from build123d import *

# Parameters (mm, degrees)
F0_R     = 3
F1_DEPTH = 50
F2_R     = 1
F3_R     = 10
F3_R_2   = 3
F4_DEPTH = 20
F5_R     = 1


with BuildPart() as f1:
    # F0 (on Front) → F1 (new body)
    with BuildSketch(Plane.XZ):
        Circle(F0_R)
    extrude(amount=F1_DEPTH)

    # F2
    f2_edges = [f1.edges().sort_by_distance(p)[0] for p in [
        (-3, 0, 0),
    ]]
    fillet(f2_edges, radius=F2_R)

    # F3 (on face) → F4 (join)
    with BuildSketch(Plane.XZ.offset(50)):
        Circle(F3_R)
        Circle(F3_R_2, mode=Mode.SUBTRACT)
    extrude(amount=-F4_DEPTH)

    # F5
    f5_edges = [f1.edges().sort_by_distance(p)[0] for p in [
        (-3, -30, 0),
        (-10, -30, 0),
        (-10, -50, 0),
    ]]
    fillet(f5_edges, radius=F5_R)


solid = f1.part
Source: CAD feature listing. Evaluate the final solid. Frame: model axes, mm. A direction names the side the tool comes from. Coordinates: 2 decimals unless noted, no trailing zeros. Loops run counter-clockwise (first coordinate to the right, second up) from the corner with the lowest first, then second, coordinate; pieces in that order, holes last. Notation, with made-up numbers: (10, 20.25) -> (27, 20.25) arc R11 cw to (27, 32.25) -> close; hole circle Ø7 at (33, -29). An arc over 180 degrees is marked (long way). Answer in a Markdown table with one row per item. Add a question column.
Q1. Ray query, line 1 along Y through (x, z) = (-8, 0.5); line 2 along X through (y, z) = (-8.5, -0.25); line 3 along X through (y, z) = (-16.5, 1.5). Return the intervals inside material, ascending.
Q2. Section D-D on y = -27. Return the cut outline in (x, z).
Q3. Pull-direction query (Y, two-part tool) for faces 3 (the face through (0, -50, 0)), 4 (the face through (2, -30, -4)), 5 (the face through (-2.17, -40.13, -9.76)); classes: pulls with the +Y half, pulls with the -Y half, needs draft (parallel to the pull), parting line crosses it, or undercut.
Q4. Section A-A on z = 0. Return the cut outline in (x, y), and give its area (3 significant figures).
Q5. Reachability of faces 1 (the face through (0, 0, 0)), 2 (the face through (-3, -15, 0)) from +Z, -Z, +X, -X, +Y, -Y: full face, straight path, thin tool, end or side. Return the list, or none.
Q6. Contact query for flat-ended pins moving along their axis: pin 1 Ø4 at (x, y) = (5.5, -29) entering from +Z; pin 2 Ø2 at (x, y) = (2.5, -17) entering from +Z; pin 3 Ø12 at (x, y) = (3.5, -38.5) entering from -Z; pin 4 Ø8 at (y, z) = (-17, -5) entering from +X. Output: stop coordinate, or through.
Q7. Section C-C on y = -37. Return the cut outline in (x, z), and give its area (3 significant figures).
Q8. Section B-B on x = 0. Return the cut outline in (y, z), and give its area (3 significant figures).
Computed values:
| question | item | result |
|---|---|---|
| 1 | line 1 | y = -50 to -30 |
| 1 | line 2 | x = -2.99 to 2.99 |
| 1 | line 3 | x = -2.6 to 2.6 |
| 2 | outline | circle Ø6 at (0, 0) |
| 3 | face 3 | pulls with the -Y half |
| 3 | face 4 | pulls with the +Y half |
| 3 | face 5 | needs draft |
| 4 | outline | (-10, -49) arc R1 ccw to (-9, -50) -> (9, -50) arc R1 ccw to (10, -49) -> (10, -31) arc R1 ccw to (9, -30) -> (4, -30) arc R1 cw to (3, -29) -> (3, -1) arc R1 ccw to (2, 0) -> (-2, 0) arc R1 ccw to (-3, -1) -> (-3, -29) arc R1 cw to (-4, -30) -> (-9, -30) arc R1 ccw to (-10, -31) -> close |
| 4 | area | 579 mm^2 |
| 5 | face 1 | +Z, -Z, +X, -X, +Y |
| 5 | face 2 | +Y |
| 6 | pin 1 | stops at z = 8.94 |
| 6 | pin 2 | stops at z = 2.6 |
| 6 | pin 3 | stops at z = -10 |
| 6 | pin 4 | stops at x = 2.83 |
| 7 | outline | circle Ø20 at (0, 0) |
| 7 | area | 314 mm^2 |
| 8 | outline | (-50, -9) arc R1 ccw to (-49, -10) -> (-31, -10) arc R1 ccw to (-30, -9) -> (-30, -4) arc R1 cw to (-29, -3) -> (-1, -3) arc R1 ccw to (0, -2) -> (0, 2) arc R1 ccw to (-1, 3) -> (-29, 3) arc R1 cw to (-30, 4) -> (-30, 9) arc R1 ccw to (-31, 10) -> (-49, 10) arc R1 ccw to (-50, 9) -> close |
| 8 | area | 579 mm^2 |
